Design review of the part built by this model. Coordinates are the model's own, in mm. Round coordinates to 2 decimals unless told otherwise and drop trailing zeros. Write each loop counter-clockwise with the first axis right and the second up, starting at its lowest first coordinate (ties: lowest second). Pieces come first, ordered by that corner, then holes. Notation, with made-up numbers: (-26.75, -29.5) -> (16.25, -29.5) arc R22 cw to (16.25, -2.5) -> close; hole circle Ø2 at (41, 81). An arc over 180 degrees is marked (long way). Write item = value, one per line. Start each with the question number.
Item 1: Add section A-A, the plane x = -2.5. State the section outline as (y, z) points (3 decimals).
Item 2: To check wall thickness, follow L1, parallel to Y at x = -4.5, z = 0 (3 decimals); L2, parallel to Y at x = 0, z = 0.5 (3 decimals); L3, parallel to Y at x = 0, z = 3.5 (3 decimals). State the ranges of each line that lie inside material, in increasing order.
Item 3: Add section D-D, the plane y = -26. State the section outline as (x, z) points (1 decimal), then the cut area to 3 significant figures.
Item 4: For pin 1 Ø1.2 at (y, z) = (-46.863, 0) entering from -X; pin 2 Ø2 at (x, y) = (-4, -52) entering from +Z, all flat-tipped, find the tip position at first contact; note any pin that passes through.
Item 5: Add section B-B, the plane z = 3. State the section outline as (x, y) points (3 decimals).
from build123d import *

# Parameters (mm, degrees)
SKETCH1_R                           = 4.7625
BOSS_EXTRUDE1_DEPTH                 = 9.525
SKETCH2_R                           = 4.7625
BOSS_EXTRUDE2_DEPTH                 = 53.34
CUT_EXTRUDE1_REACH                  = 65.225
CUT_EXTRUDE1_END_RADIUS             = 4.7625
SKETCH3_R                           = 1.0414
CUT_EXTRUDE1_DIRECTION_2_REACH      = 65.225
CUT_EXTRUDE1_DIRECTION_2_END_RADIUS = 4.7625
CUT_EXTRUDE2_REACH                  = 65.225
CUT_EXTRUDE2_END_RADIUS             = 4.7625
SKETCH4_R                           = 1.0414
CUT_EXTRUDE2_DIRECTION_2_REACH      = 65.225
CUT_EXTRUDE2_DIRECTION_2_END_RADIUS = 4.7625


with BuildPart() as part:
    # Sketch1 → Boss-Extrude1 (new body)
    with BuildSketch(Plane(origin=(0, 0, 0), x_dir=(1, 0, 0), z_dir=(0, 1, 0))):
        with Locations(Location((0, 0, 0), (0, 0, 270))):
            Circle(SKETCH1_R)
    extrude(amount=-BOSS_EXTRUDE1_DEPTH)

    # Sketch2 → Boss-Extrude2 (add)
    with BuildSketch(Plane(origin=(0, -9.525, 0), x_dir=(-1, 0, 0), z_dir=(0, -1, 0))):
        with Locations(Location((0, 0, 0), (0, 0, 270))):
            Circle(SKETCH2_R)
    extrude(amount=BOSS_EXTRUDE2_DEPTH)

    # Cut-Extrude1: up to this cylinder (the profile starts inside it)
    cut_extrude1_end = Plane(origin=(0, -5.08, 0), z_dir=(0, 1, 0)) * Cylinder(CUT_EXTRUDE1_END_RADIUS, 140.975, mode=Mode.PRIVATE)
    # Sketch3 → Cut-Extrude1 (cut, up to the surface)
    with BuildSketch(Plane.XY, mode=Mode.PRIVATE) as cut_extrude1_sk1:
        with Locations((0, -5.08)):
            Circle(SKETCH3_R)
    cut_extrude1_tool1 = extrude(cut_extrude1_sk1.sketch, amount=-CUT_EXTRUDE1_REACH, mode=Mode.PRIVATE) & cut_extrude1_end
    add(cut_extrude1_tool1.solids().sort_by_distance((0, -5.08, 0))[0], mode=Mode.SUBTRACT)

    # Cut-Extrude1 direction 2: up to this cylinder (the profile starts inside it)
    cut_extrude1_direction_2_end = Plane(origin=(0, -5.08, 0), z_dir=(0, 1, 0)) * Cylinder(CUT_EXTRUDE1_DIRECTION_2_END_RADIUS, 140.975, mode=Mode.PRIVATE)
    # Sketch3 → Cut-Extrude1 direction 2 (cut, up to the surface)
    with BuildSketch(Plane.XY, mode=Mode.PRIVATE) as cut_extrude1_direction_2_sk1:
        with Locations((0, -5.08)):
            Circle(SKETCH3_R)
    cut_extrude1_direction_2_tool1 = extrude(cut_extrude1_direction_2_sk1.sketch, amount=CUT_EXTRUDE1_DIRECTION_2_REACH, mode=Mode.PRIVATE) & cut_extrude1_direction_2_end
    add(cut_extrude1_direction_2_tool1.solids().sort_by_distance((0, -5.08, 0))[0], mode=Mode.SUBTRACT)

    # Cut-Extrude2: up to this cylinder (the profile starts inside it)
    cut_extrude2_end = Plane(origin=(0, -46.863, 0), z_dir=(0, 1, 0)) * Cylinder(CUT_EXTRUDE2_END_RADIUS, 140.975, mode=Mode.PRIVATE)
    # Sketch4 → Cut-Extrude2 (cut, up to the surface)
    with BuildSketch(Plane(origin=(0, 0, 0), x_dir=(0, 0, -1), z_dir=(1, 0, 0)), mode=Mode.PRIVATE) as cut_extrude2_sk1:
        with Locations((0, -46.863)):
            Circle(SKETCH4_R)
    cut_extrude2_tool1 = extrude(cut_extrude2_sk1.sketch, amount=-CUT_EXTRUDE2_REACH, mode=Mode.PRIVATE) & cut_extrude2_end
    add(cut_extrude2_tool1.solids().sort_by_distance((0, -46.863, 0))[0], mode=Mode.SUBTRACT)

    # Cut-Extrude2 direction 2: up to this cylinder (the profile starts inside it)
    cut_extrude2_direction_2_end = Plane(origin=(0, -46.863, 0), z_dir=(0, 1, 0)) * Cylinder(CUT_EXTRUDE2_DIRECTION_2_END_RADIUS, 140.975, mode=Mode.PRIVATE)
    # Sketch4 → Cut-Extrude2 direction 2 (cut, up to the surface)
    with BuildSketch(Plane(origin=(0, 0, 0), x_dir=(0, 0, -1), z_dir=(1, 0, 0)), mode=Mode.PRIVATE) as cut_extrude2_direction_2_sk1:
        with Locations((0, -46.863)):
            Circle(SKETCH4_R)
    cut_extrude2_direction_2_tool1 = extrude(cut_extrude2_direction_2_sk1.sketch, amount=CUT_EXTRUDE2_DIRECTION_2_REACH, mode=Mode.PRIVATE) & cut_extrude2_direction_2_end
    add(cut_extrude2_direction_2_tool1.solids().sort_by_distance((0, -46.863, 0))[0], mode=Mode.SUBTRACT)


solid = part.part
Result set:
q1.outline = (-62.865, -4.054) -> (0, -4.054) -> (0, 4.054) -> (-62.865, 4.054) -> close; hole circle Ø2.083 at (-46.863, 0)
q2.L1 = -62.865 to -47.904, -45.822 to 0
q2.L2 = -62.865 to -47.777, -45.949 to -6.121, -4.039 to 0
q2.L3 = -62.865 to -6.121, -4.039 to 0
q3.outline = circle Ø9.5 at (0, 0)
q3.area = 71.3 mm²
q4.pin_1 = through
q4.pin_2 = 3.7
q5.outline = (-3.699, -62.865) -> (3.699, -62.865) -> (3.699, 0) -> (-3.699, 0) -> close; hole circle Ø2.083 at (0, -5.08)
